Geometry check sheet. Reference: drawing and pictorial views, mm from the part's lowest x, y, z. A direction names the side the tool comes from. Round coordinates to 2 decimals unless told otherwise and drop trailing zeros. Write each loop counter-clockwise with the first axis right and the second up, starting at its lowest first coordinate (ties: lowest second). Pieces come first, ordered by that corner, then holes. Notation, with made-up numbers: M 5.5,29.25 L 22.5,29.25 A14 ccw 22.5,33.25 Z; hole C -26,-9 d5. An arc over 180 degrees is marked long. Answer in a Markdown table with one row per item. Add a question column.
1. Go/stop test with flat-tipped pins: pin 1 Ø10 at (x, z) = (23.5, 24) entering from +Y; pin 2 Ø3 at (y, z) = (55.5, 61.5) entering from -X; pin 3 Ø6 at (x, z) = (37, 79.5) entering from +Y; pin 4 Ø8 at (x, z) = (74, 42) entering from -Y. Record where each tip stops, or that it passes through.
2. Sectioned sample at A-A on x = 11.5. Record the cut outline in (y, z), plus the area to 3 significant figures.
3. Sectioned sample at B-B on y = 45.05. Count the separate pieces of the cut face and the enclosed holes in it, plus the area to 3 significant figures.
4. Draft check along Z on the marked faces 1, 2 and 3. Enter one of: pulls with the +Z half, pulls with the -Z half, needs draft (parallel to the pull), parting line crosses it, or undercut.
5. Material ranges on probe 1 along X at (y, z) = (77, 45.05), recorded low to high.
6. Set-up check for the marked faces 4, 5, 6 and 7: record each of +Z, -Z, +X, -X, +Y, -Y from which the full face is reachable in a straight line by a thin tool's end or side.
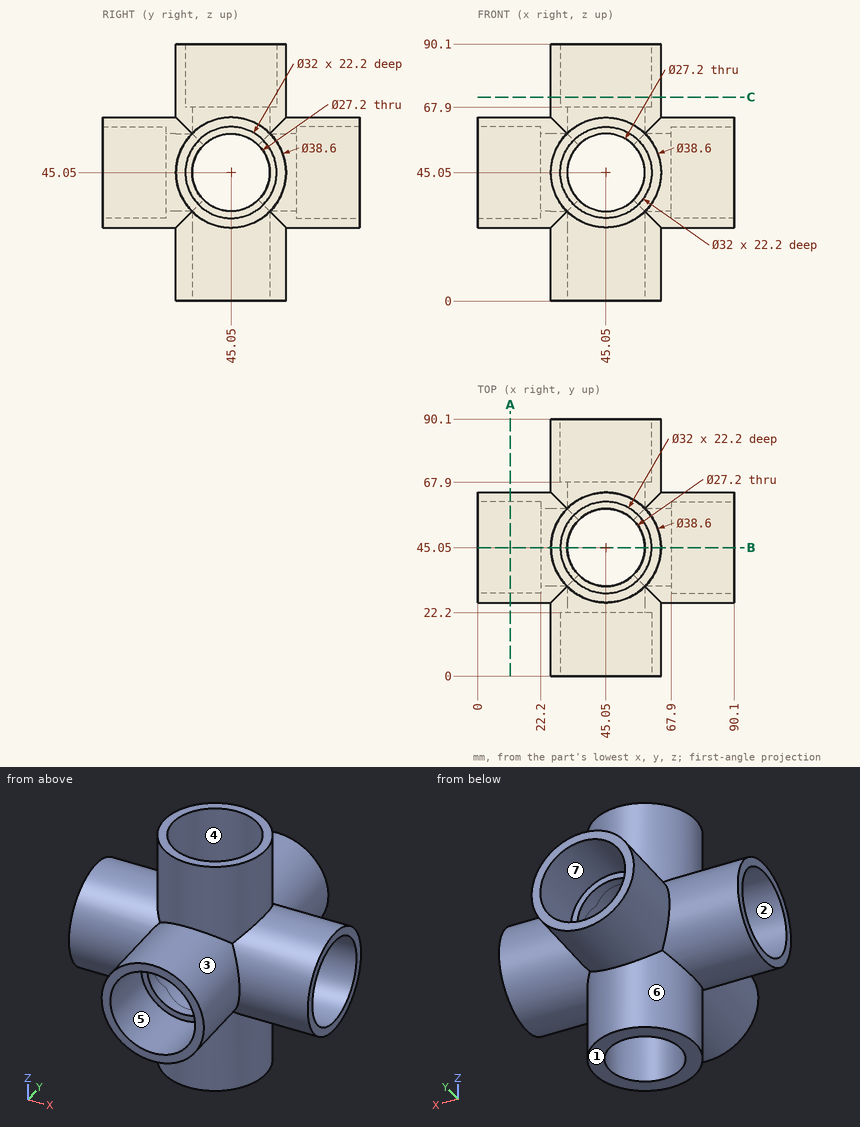
Geometry check:
| question | item | result |
|---|---|---|
| 1 | pin 1 | stops at y = 55.77 |
| 1 | pin 2 | stops at x = 0 |
| 1 | pin 3 | stops at y = 63.68 |
| 1 | pin 4 | stops at y = 25.75 |
| 2 | outline | C 45.05,45.05 d38.6; hole C 45.05,45.05 d32 |
| 2 | area | 366 mm2 |
| 3 | separate pieces | 4 |
| 3 | enclosed holes | 0 |
| 3 | area | 984 mm2 |
| 4 | face 1 | pulls with the -Z half |
| 4 | face 2 | undercut |
| 4 | face 3 | parting line crosses it |
| 5 | probe 1 | x = 25.75 to 29.05, 61.05 to 64.35 |
| 6 | face 4 | +Z |
| 6 | face 5 | -Y |
| 6 | face 6 | -Z |
| 6 | face 7 | +Y |
